from build123d import *

# Parameters (mm, degrees)
SKETCH1_R           = 50
BOSS_EXTRUDE1_DEPTH = 45
BOSS_EXTRUDE2_START = 5
SKETCH2_R           = 50
BOSS_EXTRUDE2_DEPTH = 5
SKETCH3_R           = 2.5
CUT_EXTRUDE1_DEPTH  = 3
SKETCH4_R           = 25
CUT_EXTRUDE2_DEPTH  = 10


with BuildPart() as part:
    # Sketch1 → Boss-Extrude1 (new body)
    with BuildSketch(Plane(origin=(0, 0, 0), x_dir=(1, 0, 0), z_dir=(0, 1, 0))):
        with Locations(Location((0, 0, 0), (0, 0, 90))):
            Circle(SKETCH1_R)
        with BuildLine():
            ThreePointArc((-38.472091197, 10.949803601), (-39.142843019, 8.236373014), (-39.622464899, 5.482725176))
            ThreePointArc((-39.622464899, 5.482725176), (-45.027736203, 0.561560709), (-39.746875, -4.492875219))
            ThreePointArc((-39.746875, -4.492875219), (-39.333953887, -7.269117664), (-38.72736158, -10.009568673))
            ThreePointArc((-38.72736158, -10.009568673), (-41.748946282, -16.583911093), (-35.039748856, -19.292900251))
            ThreePointArc((-35.039748856, -19.292900251), (-33.590491244, -21.718169766), (-31.973653194, -24.035088963))
            ThreePointArc((-31.973653194, -24.035088963), (-32.157729031, -31.176050772), (-25.014492656, -31.213381059))
            ThreePointArc((-25.014492656, -31.213381059), (-22.728868069, -32.915020223), (-20.32789937, -34.449622744))
            ThreePointArc((-20.32789937, -34.449622744), (-17.707258167, -40.991172437), (-11.148020432, -38.415122549))
            ThreePointArc((-11.148020432, -38.415122549), (-8.358901204, -39.11686044), (-5.526568431, -39.6163734))
            ThreePointArc((-5.526568431, -39.6163734), (-0.59402965, -44.528471783), (4.46778962, -39.749702589))
            ThreePointArc((4.46778962, -39.749702589), (7.33562934, -39.321604013), (10.164921368, -38.686875986))
            ThreePointArc((10.164921368, -38.686875986), (16.574401115, -41.242300251), (19.433073291, -34.962203341))
            ThreePointArc((19.433073291, -34.962203341), (21.927230073, -33.454395546), (24.304976528, -31.768980405))
            ThreePointArc((24.304976528, -31.768980405), (31.177616874, -31.629495833), (31.415975195, -24.759573957))
            ThreePointArc((31.415975195, -24.759573957), (33.136656406, -22.404508524), (34.681152562, -19.930320042))
            ThreePointArc((34.681152562, -19.930320042), (40.985236081, -17.155873875), (38.537324177, -10.717959006))
            ThreePointArc((38.537324177, -10.717959006), (39.213686022, -7.892200491), (39.683137427, -5.024798895))
            ThreePointArc((39.683137427, -5.024798895), (44.500790375, -0.031685054), (39.690252613, 4.968284165))
            ThreePointArc((39.690252613, 4.968284165), (39.229069194, 7.815377799), (38.563928149, 10.62183815))
            ThreePointArc((38.563928149, 10.62183815), (41.191547229, 17.128956276), (34.724740733, 19.854278657))
            ThreePointArc((34.724740733, 19.854278657), (33.21843503, 22.283078202), (31.542548716, 24.598122296))
            ThreePointArc((31.542548716, 24.598122296), (31.568070741, 31.71029047), (24.456089141, 31.652799306))
            ThreePointArc((24.456089141, 31.652799306), (22.154728904, 33.304173721), (19.742272443, 34.788542349))
            ThreePointArc((19.742272443, 34.788542349), (17.102427339, 41.494962196), (10.503764758, 38.596255335))
            ThreePointArc((10.503764758, 38.596255335), (7.766185163, 39.238837496), (4.99022482, 39.6875))
            ThreePointArc((4.99022482, 39.6875), (0, 45), (-4.99022482, 39.6875))
            ThreePointArc((-4.99022482, 39.6875), (-7.752560801, 39.241531584), (-10.476960655, 38.603539934))
            ThreePointArc((-10.476960655, 38.603539934), (-17.137978748, 41.698652845), (-19.697351689, 34.813996272))
            ThreePointArc((-19.697351689, 34.813996272), (-22.077028029, 33.355731643), (-24.349225183, 31.735078903))
            ThreePointArc((-24.349225183, 31.735078903), (-31.708929174, 32.096652706), (-31.436823309, 24.733098071))
            ThreePointArc((-31.436823309, 24.733098071), (-33.084428294, 22.481561432), (-34.571077134, 20.120651724))
            ThreePointArc((-34.571077134, 20.120651724), (-41.501374638, 17.653486782), (-38.472091197, 10.949803601))
        make_face(mode=Mode.SUBTRACT)
    extrude(amount=BOSS_EXTRUDE1_DEPTH)

    # Sketch2 → Boss-Extrude2 (add)
    with BuildSketch(Plane.XZ.offset(BOSS_EXTRUDE2_START)):
        with Locations(Location((0, 0, 0), (0, 0, 270))):
            Circle(SKETCH2_R)
    extrude(amount=-BOSS_EXTRUDE2_DEPTH)

    # Sketch3 → Cut-Extrude1 (cut)
    with BuildSketch(Plane(origin=(0, 0, 0), x_dir=(1, 0, 0), z_dir=(0, 1, 0))):
        with Locations(Location((0, 40, 0), (0, 0, 270))):
            Circle(SKETCH3_R)
        with Locations(Location((15.307337295, 36.9551813, 0), (0, 0, 270))):
            Circle(SKETCH3_R)
        with Locations(Location((28.284271247, 28.284271247, 0), (0, 0, 270))):
            Circle(SKETCH3_R)
        with Locations(Location((36.9551813, 15.307337295, 0), (0, 0, 270))):
            Circle(SKETCH3_R)
        with Locations(Location((40, 0, 0), (0, 0, 270))):
            Circle(SKETCH3_R)
        with Locations(Location((36.9551813, -15.307337295, 0), (0, 0, 270))):
            Circle(SKETCH3_R)
        with Locations(Location((28.284271247, -28.284271247, 0), (0, 0, 270))):
            Circle(SKETCH3_R)
        with Locations(Location((15.307337295, -36.9551813, 0), (0, 0, 270))):
            Circle(SKETCH3_R)
        with Locations(Location((0, -40, 0), (0, 0, 270))):
            Circle(SKETCH3_R)
        with Locations(Location((-15.307337295, -36.9551813, 0), (0, 0, 270))):
            Circle(SKETCH3_R)
        with Locations(Location((-28.284271247, -28.284271247, 0), (0, 0, 270))):
            Circle(SKETCH3_R)
        with Locations(Location((-36.9551813, -15.307337295, 0), (0, 0, 270))):
            Circle(SKETCH3_R)
        with Locations(Location((-40, 0, 0), (0, 0, 270))):
            Circle(SKETCH3_R)
        with Locations(Location((-36.9551813, 15.307337295, 0), (0, 0, 270))):
            Circle(SKETCH3_R)
        with Locations(Location((-28.284271247, 28.284271247, 0), (0, 0, 270))):
            Circle(SKETCH3_R)
        with Locations(Location((-15.307337295, 36.9551813, 0), (0, 0, 270))):
            Circle(SKETCH3_R)
    extrude(amount=-CUT_EXTRUDE1_DEPTH, mode=Mode.SUBTRACT)

    # Sketch4 → Cut-Extrude2 (cut)
    with BuildSketch(Plane(origin=(0, 0, 0), x_dir=(1, 0, 0), z_dir=(0, 1, 0))):
        with Locations(Location((0, 0, 0), (0, 0, 270))):
            Circle(SKETCH4_R)
    extrude(amount=-CUT_EXTRUDE2_DEPTH, mode=Mode.SUBTRACT)


solid = part.part
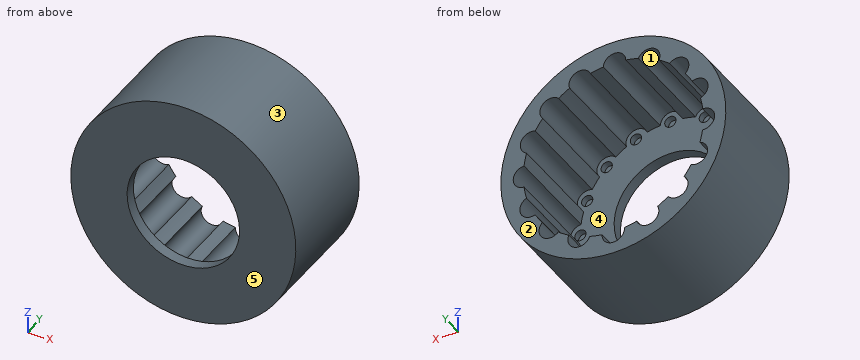
Build history of the part. All positions in model axes, mm. Face numbers are marked on the shaded views. A direction names the side the tool comes from. Round coordinates to 2 decimals unless told otherwise and drop trailing zeros. Loops run counter-clockwise (first coordinate to the right, second up) from the corner with the lowest first, then second, coordinate; pieces in that order, holes last. Notation, with made-up numbers: (61.5, 62) -> (82.5, 62) arc R4 ccw to (82.5, 67) -> close; hole circle Ø1 at (-34, 85.5). An arc over 180 degrees is marked (long way). One line per item, written item: value. Start each with the question number.
Q1. 3-axis set-ups, long thin cutter, end or side, ignore diameter. For the marked faces 1 and 2: which of +Z, -Z, +X, -X, +Y, -Y reach the whole face in a straight line?
Q2. Drop flat-ended pins along their axis: pin 1 Ø5.5 at (x, z) = (16.5, -37.5) entering from +Y; pin 2 Ø1.5 at (x, z) = (-16.5, -37) entering from +Y; pin 3 Ø8 at (x, y) = (-30, 36.5) entering from -Z; pin 4 Ø5 at (x, y) = (0.5, 38) entering from +Z. Give the stop position or say it passes through.
Q3. Probe line 1 along Z through (x, y) = (-32.5, 21); line 2 along Y through (x, z) = (32, 5.5); line 3 along X through (y, z) = (17, 23). List the from-to ranges inside material, lowest first.
Q4. Cut at B-B on z = -16. List the corners of the cut face in (x, y).
Q5. Two-plate mould, pull along Z, no slides. Class the marked faces 3, 4 and 5: released by +Z, released by -Z, zero draft, split by the parting line, or undercut.
Q6. Cut at C-C on x = 0. List the corners of the cut face in (y, z), plus the area to 3 significant figures.
Computed:
1. face 1: +Y
1. face 2: +Z, -Z, +X, -X, +Y
2. pin 1: y = 0
2. pin 2: y = -3
2. pin 3: z = -42.71
2. pin 4: z = 50
3. line 1: -38 to -31.08, -26 to -23.32, 23.32 to 24.61, 30.78 to 38
3. line 2: -5 to 0
3. line 3: -44.4 to -32.73, 32.73 to 44.4
4. outline: (-47.37, -5) -> (-19.21, -5) -> (-19.21, 0) -> (-34.55, 0) -> (-34.55, -3) -> (-39.36, -3) -> (-39.36, 0) -> (-41.89, 0) -> (-41.89, 45) -> (-47.37, 45) -> close; (19.21, -5) -> (47.37, -5) -> (47.37, 45) -> (41.51, 45) -> (41.51, 0) -> (39.36, 0) -> (39.36, -3) -> (34.55, -3) -> (34.55, 0) -> (19.21, 0) -> close
5. face 3: split by the parting line
5. face 4: undercut
5. face 5: zero draft
6. outline: (-5, -50) -> (45, -50) -> (45, -45) -> (0, -45) -> (0, -42.5) -> (-3, -42.5) -> (-3, -37.5) -> (0, -37.5) -> (0, -25) -> (-5, -25) -> close; (-5, 25) -> (0, 25) -> (0, 37.5) -> (-3, 37.5) -> (-3, 42.5) -> (0, 42.5) -> (0, 44.5) -> (45, 44.5) -> (45, 50) -> (-5, 50) -> close
6. area: 692 mm²
